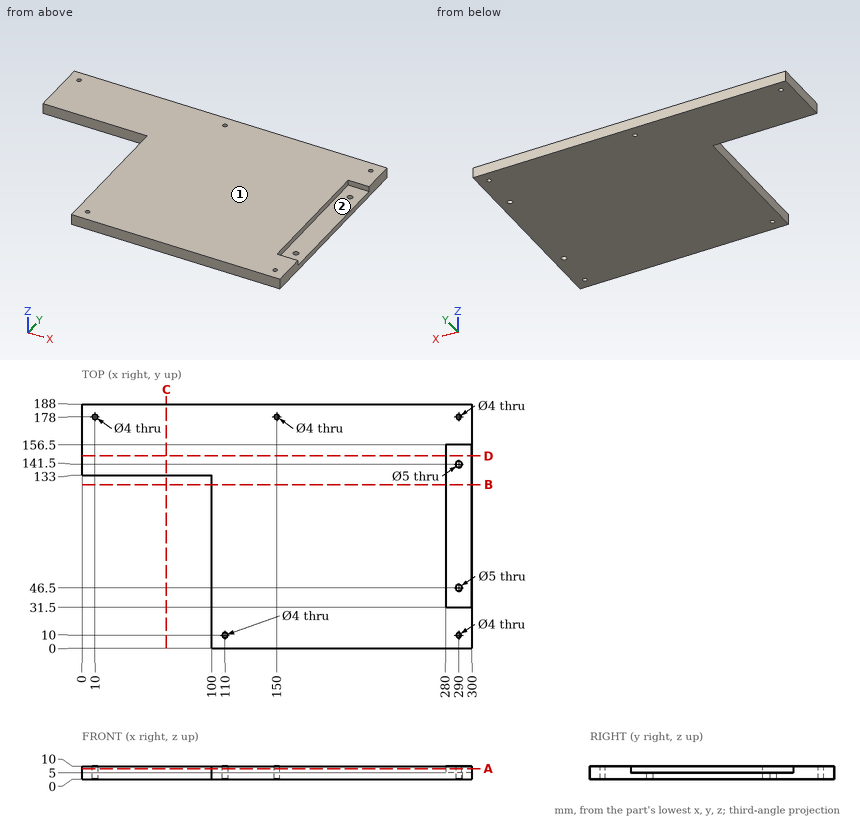
Here's the drawing with two shaded views (mm, measured from the low corner). I have some questions. Give positions to 0.01 mm unless a question says otherwise; leave off trailing zeros. Order: outer loops, then holes, each group sorted by start corner. A loop starts at its lowest first (then second) coordinate and runs counter-clockwise, first axis right, second up.
Q1. I'm going to push flat-ended pins straight in: P1, Ø6, axis at x = 286.5, y = 120.5, coming from the +Z side; P2, Ø3, axis at y = 97.5, z = 4, coming from the -X side; P3, Ø2.5, axis at y = 96.5, z = 8, coming from the +X side. Where does each tip first touch, or does it pass through?
Q2. Suppose I cut it at B-B, the plane y = 126. Write out the boundary of the cut face in (x, z).
Q3. Suppose I cut it at C-C, the plane x = 65. Write out the boundary of the cut face in (y, z).
Q4. We'd pull the mould along Y, two halves only. Please class the marked faces 1 and 2: +Y half, -Y half, draft (parallel to the pull), parting line (faces both ways), or undercut.
Q5. Suppose I cut it at A-A, the plane z = 8.25. Write out the boundary of the cut face in (x, y).
Q6. If I drill on line 1 along Y through (x, z) = (290, 7.75); line 2 along X through (y, z) = (178, 5); line 3 along Y through (x, z) = (110, 3.5), over which ranges is the centre line in solid material (lowest first)?
Q7. Suppose I cut it at D-D, the plane y = 148. Write out the boundary of the cut face in (x, z), and give its area (3 significant figures).
Solution:
1. P1: stops at z = 5
1. P2: stops at x = 100
1. P3: stops at x = 280
2. outline: (100, 0) - (300, 0) - (300, 5) - (280, 5) - (280, 10) - (100, 10) - close
3. outline: (133, 0) - (188, 0) - (188, 10) - (133, 10) - close
4. face 1: draft
4. face 2: undercut
5. outline: (0, 133) - (100, 133) - (100, 0) - (300, 0) - (300, 31.5) - (280, 31.5) - (280, 156.5) - (300, 156.5) - (300, 188) - (0, 188) - close; hole circle Ø4 at (10, 178); hole circle Ø4 at (110, 10); hole circle Ø4 at (150, 178); hole circle Ø4 at (290, 10); hole circle Ø4 at (290, 178)
6. line 1: y = 0 to 8, 12 to 31.5, 156.5 to 176, 180 to 188
6. line 2: x = 0 to 8, 12 to 148, 152 to 288, 292 to 300
6. line 3: y = 0 to 8, 12 to 188
7. outline: (0, 0) - (300, 0) - (300, 5) - (280, 5) - (280, 10) - (0, 10) - close
7. area: 2,900 mm2
